Could you check a few things on this drawing? It's one solid part, dimensions in mm from its lowest x, y, z. Coordinates: 2 decimals unless noted, no trailing zeros. Write each loop counter-clockwise with the first axis right and the second up, starting at its lowest first coordinate (ties: lowest second). Pieces come first, ordered by that corner, then holes. Notation, with made-up numbers: (35, -7) - (62, -7) arc R33 cw to (62, 30) - close; hole circle Ø7 at (37, 62.25). An arc over 180 degrees is marked (long way). Use one line per item in the form item = value. Start each with the question number.
(1) If we section it at C-C on z = 159: Please give me the cut outline in (x, y).
(2) Thinking about a two-plate mould opening in X: for the marked faces 1, 2 and 3, which applies, pulls with the +X half, pulls with the -X half, needs draft (parallel to the pull), parting line crosses it, or undercut?
(3) If I drill on probe 1 along Y at (x, z) = (80, 2); probe 2 along Z at (x, y) = (141, 76); probe 3 along Z at (x, y) = (99.5, 75.5), over which ranges is the centre line in solid material (lowest first)? Write a range as from..to.
(4) If we section it at A-A on x = 80: Please give me the cut outline in (y, z), then the cut area to 3 significant figures.
(5) For pin 1 Ø1.5 at (x, z) = (25, 93) entering from +Y; pin 2 Ø2 at (x, z) = (87.5, 75.5) entering from +Y; pin 3 Ø10 at (x, z) = (45.5, 117) entering from -Y, each with a flat end and sliding along its axis, tell me the tip position at first contact or that it passes through.
(6) If we section it at D-D on y = 119: Please give me the cut outline in (x, z), then the cut area to 3 significant figures.
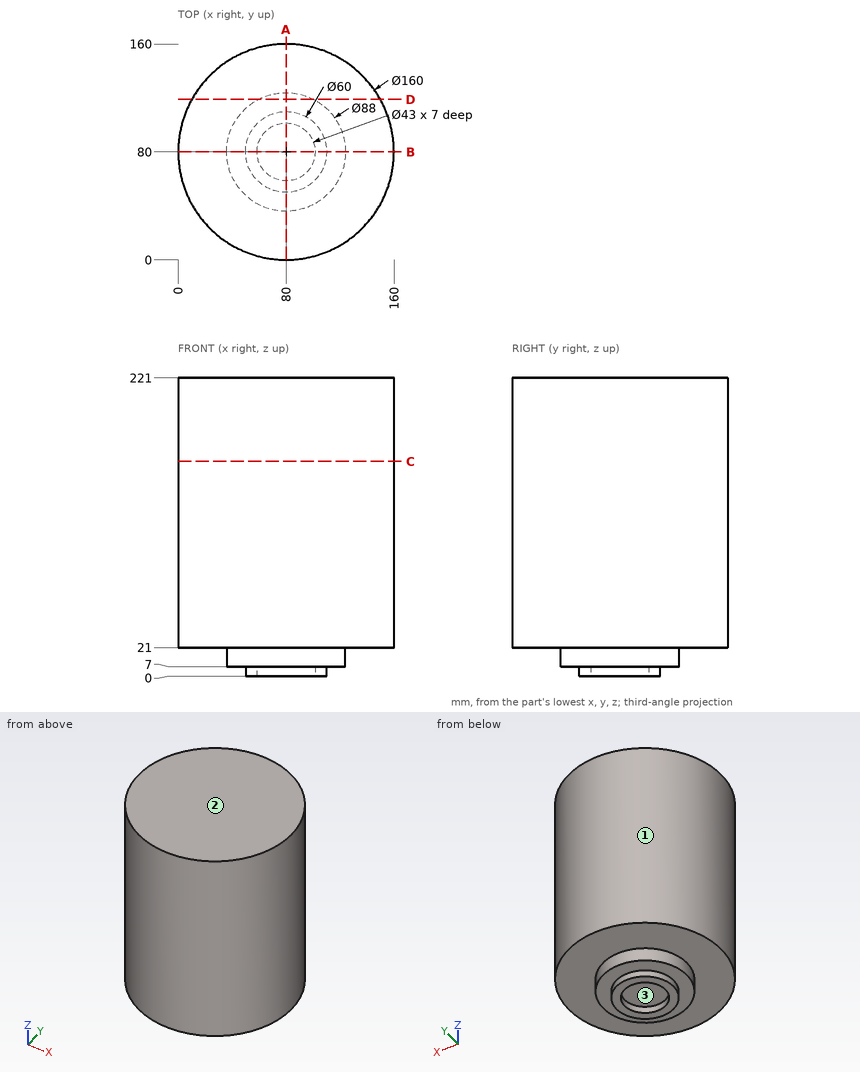
Reported:
q1.outline = circle Ø160 at (80, 80)
q2.face_1 = parting line crosses it
q2.face_2 = needs draft
q2.face_3 = undercut
q3.probe_1 = 50..58.5, 101.5..110
q3.probe_2 = 21..221
q3.probe_3 = 7..221
q4.outline = (0, 21) - (36, 21) - (36, 7) - (50, 7) - (50, 0) - (58.5, 0) - (58.5, 7) - (101.5, 7) - (101.5, 0) - (110, 0) - (110, 7) - (124, 7) - (124, 21) - (160, 21) - (160, 221) - (0, 221) - close
q4.area = 33,400 mm2
q5.pin_1 = 138.8
q5.pin_2 = 159.74
q5.pin_3 = 5.64
q6.outline = (10.15, 21) - (59.63, 21) - (59.63, 7) - (100.37, 7) - (100.37, 21) - (149.85, 21) - (149.85, 221) - (10.15, 221) - close
q6.area = 28,500 mm2
